Could you check a few things on this drawing? It's one solid part, dimensions in mm from its lowest x, y, z. A direction names the side the tool comes from. Round coordinates to 2 decimals unless told otherwise and drop trailing zeros. Order: outer loops, then holes, each group sorted by start corner. A loop starts at its lowest first (then second) coordinate and runs counter-clockwise, first axis right, second up.
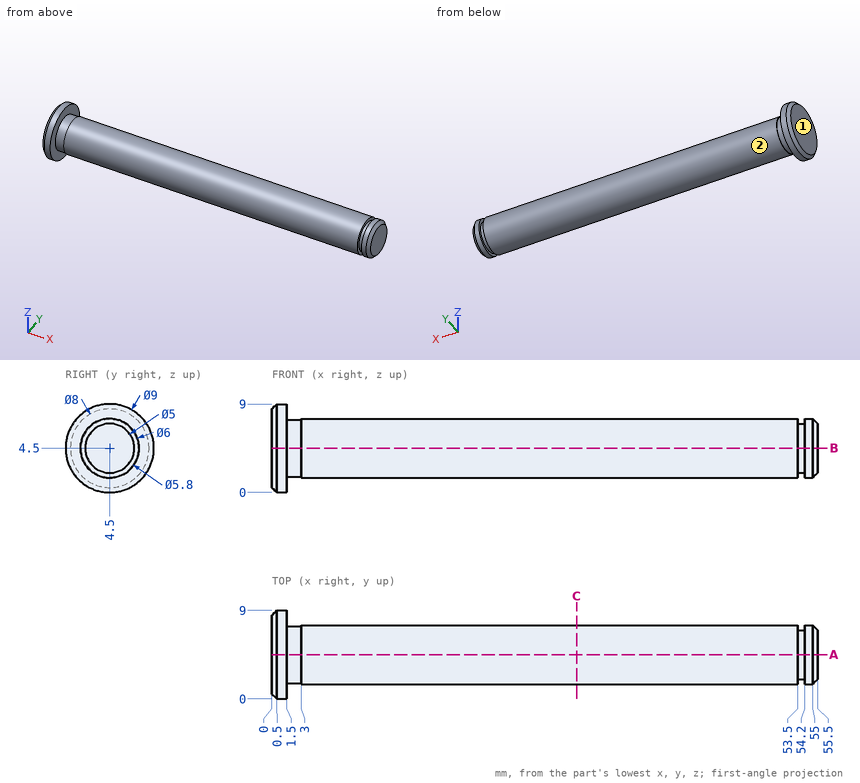
1) If we section it at A-A (y = 4.5): Write out the boundary of the cut face in (x, z).
2) If we section it at C-C (x = 31): Write out the boundary of the cut face in (y, z).
3) I need wall thicknesses on line 1 (Z direction, x = 4, y = 5.25); line 2 (X direction, y = 1.25, z = 6.5). Which ranges of each line are inside material? Lowest first, please.
4) I'm going to push flat-ended pins straight in: pin 1 (3 mm diameter, centred on x = 12, z = 6, fed in from -Y); pin 2 (1 mm diameter, centred on x = 39.5, y = 2.5, fed in from -Z); pin 3 (1 mm diameter, centred on x = 12.5, y = 2, fed in from -Z). Where does each tip first touch, or does it pass through?
5) For the marked faces 1 and 2, which set-ups out of +Z, -Z, +X, -X, +Y, -Y let a thin tool reach every point of the face, with its end or its side?
Solutions:
1. outline: (0, 0.5) - (0.5, 0) - (1.5, 0) - (1.5, 1.6) - (3, 1.6) - (3, 1.5) - (53.5, 1.5) - (53.5, 2) - (54.2, 2) - (54.2, 1.5) - (55, 1.5) - (55.5, 2) - (55.5, 7) - (55, 7.5) - (54.2, 7.5) - (54.2, 7) - (53.5, 7) - (53.5, 7.5) - (3, 7.5) - (3, 7.4) - (1.5, 7.4) - (1.5, 9) - (0.5, 9) - (0, 8.5) - close
2. outline: circle Ø6 at (4.5, 4.5)
3. line 1: z = 1.6 to 7.4
3. line 2: x = 0 to 1.5
4. pin 1: stops at y = 1.5
4. pin 2: stops at z = 1.9
4. pin 3: stops at z = 2.26
5. face 1: +Z, -Z, -X, +Y, -Y
5. face 2: +X
